from build123d import *

# Parameters (mm, degrees)
EXTRUDE_1_DEPTH      = 80
EXTRUDE_1_DEPTH_BACK = 80
EXTRUDE_2_DEPTH      = 32
EXTRUDE_2_DEPTH_BACK = 32
CUT_EXTRUDE_6_DEPTH  = 33.957985297
CUT_EXTRUDE_START    = -22
SKETCH_14_W          = 51
SKETCH_14_H          = 3
CUT_EXTRUDE_7_DEPTH  = 98.020555692


# Read off the part's stored shape, not the designer's step: Вырез-Вытянуть6
with BuildPart() as part:
    # Эскиз11 → Бобышка-Вытянуть1 (new, two sides: drawn at the far end of the back side and taken through both)
    with BuildSketch(Plane.XY.offset(-EXTRUDE_1_DEPTH_BACK)):
        Polygon((0, 0), (33.957985297, 80), (6.999093082, 80), align=None)
    extrude(amount=EXTRUDE_1_DEPTH + EXTRUDE_1_DEPTH_BACK)

    # Эскиз13 → Бобышка-Вытянуть2 (add, two sides: drawn at the far end of the back side and taken through both)
    with BuildSketch(Plane.XY.offset(-EXTRUDE_2_DEPTH_BACK)):
        Polygon((6.999093082, 80), (-3, 4), (0, 0), align=None)
    extrude(amount=EXTRUDE_2_DEPTH + EXTRUDE_2_DEPTH_BACK)

    # Вырез-Вытянуть6 outline → Вырез-Вытянуть6 (cut)
    with BuildSketch(Plane(origin=(0, 0, 0), x_dir=(0, 0, -1), z_dir=(1, 0, 0))):
        with BuildLine():
            Line((-80, 80), (-80, 0))
            ThreePointArc((-80, 0), (-56.568542382, 56.568542608), (3.2e-07, 80))
            Line((3.2e-07, 80), (-80, 80))
        make_face()
        with BuildLine():
            ThreePointArc((3.2e-07, 80), (56.568542608, 56.568542382), (80, 0))
            Line((80, 0), (80, 80))
            Line((80, 80), (3.2e-07, 80))
        make_face()
    extrude(amount=CUT_EXTRUDE_6_DEPTH, mode=Mode.SUBTRACT)

    # Эскиз14 → Вырез-Вытянуть7 (cut, through all)
    with BuildSketch(Plane(origin=(33.957985297, 0, 0), x_dir=(0, 0, -1), z_dir=(1, 0, 0)).offset(CUT_EXTRUDE_START)):
        with Locations((0, 71.5)):
            Rectangle(SKETCH_14_W, SKETCH_14_H)
        with Locations((0, 65.5)):
            Rectangle(SKETCH_14_W, SKETCH_14_H)
    extrude(amount=-CUT_EXTRUDE_7_DEPTH, mode=Mode.SUBTRACT)


solid = part.part
The model under review builds one solid part; all positions refer to its coordinate system, in mm. A direction names the side the tool comes from. Give positions to 0.01 mm unless a question says otherwise; leave off trailing zeros. Order: outer loops, then holes, each group sorted by start corner. A loop starts at its lowest first (then second) coordinate and runs counter-clockwise, first axis right, second up. Notation, with made-up numbers: M -21.75,72 L 26.25,72 A22 ccw 26.25,101 Z; hole C 8,56 d10. An arc over 180 degrees is marked long. Answer in a Markdown table with one row per item. Add a question column.
1. Add section A-A on x = 9.5. State the section outline as (y, z) points, plus the area to 3 significant figures.
2. Machinability: for faces 1 (the flat face through (1, 26, -32)), 2 (the flat face through (2.54, 29.03, 50.33)), 3 (the flat face through (9, 71, -25.5)), which of the approach directions +Z, -Z, +X, -X, +Y, -Y give a long, thin tool a straight path to every point of the face, cutting with its end or side? Answer none if there is none.
3. Add section D-D on x = 23. State the section outline as (y, z) points, plus the area to 3 significant figures.
4. For pin 1 Ø2.5 at (x, y) = (9, 65) entering from +Z; pin 2 Ø3 at (x, z) = (10.5, 0) entering from -Y; pin 3 Ø1.5 at (y, z) = (65, -0.5) entering from -X, all flat-tipped, find the tip position at first contact; note any pin that passes through.
5. Add section B-B on y = 41.5. State the section outline as (x, z) points, plus the area to 3 significant figures.
6. Add section C-C on z = 15.5. State the section outline as (x, y) points.
7. To check wall thickness, follow line 1 along Y through (x, z) = (6, 15); line 2 along Z through (x, y) = (-0.5, 4); line 3 along X through (y, z) = (53.5, 20.5). State the ranges of each line that lie inside material, in increasing order.
8. Mouldability with a two-part tool opening along Y and no side actions: class faces 4 (the flat face through (2.07, 42.53, -0.45)), 5 (the flat face through (1, 26, 32)), 6 (the flat face through (8, 64, 0)) as released by +Y, released by -Y, zero draft, split by the parting line, or undercut.
The answers:
| question | item | result |
|---|---|---|
| 1 | outline | M 22.38,-76.81 A80 ccw 22.38,76.81 Z; hole M 64,-25.5 L 67,-25.5 L 67,25.5 L 64,25.5 Z; hole M 70,-25.5 L 73,-25.5 L 73,25.5 L 70,25.5 Z |
| 1 | area | 6,210 mm2 |
| 2 | face 1 | -Z, -X, +Y |
| 2 | face 2 | +Z, -X, +Y |
| 2 | face 3 | -X |
| 3 | outline | M 54.18,-58.86 A80 ccw 54.18,58.86 Z |
| 3 | area | 2,100 mm2 |
| 4 | pin 1 | z = 48.33 |
| 4 | pin 2 | y = 21.2 |
| 4 | pin 3 | x = 11.96 |
| 5 | outline | M 1.93,-32 L 3.63,-32 L 3.63,-68.39 L 17.62,-68.39 L 17.62,68.39 L 3.63,68.39 L 3.63,32 L 1.93,32 Z |
| 5 | area | 2,020 mm2 |
| 6 | outline | M -3,4 L 0,0 L 33.31,78.48 L 6.8,78.48 L 6.08,73 L 11.96,73 L 11.96,70 L 5.68,70 L 5.29,67 L 11.96,67 L 11.96,64 L 4.89,64 Z |
| 7 | line 1 | 14.14 to 64, 67 to 70 |
| 7 | line 2 | -32 to 32 |
| 7 | line 3 | 3.51 to 22.71 |
| 8 | face 4 | released by +Y |
| 8 | face 5 | zero draft |
| 8 | face 6 | undercut |
